Verification items for the finished model (mm, model axes). Face numbers are marked on the shaded views. A direction names the side the tool comes from. Give positions to 0.01 mm unless a question says otherwise; leave off trailing zeros. Order: outer loops, then holes, each group sorted by start corner. A loop starts at its lowest first (then second) coordinate and runs counter-clockwise, first axis right, second up. Notation, with made-up numbers: M -15.75,24.25 L 23.25,24.25 A35 ccw 23.25,63.25 Z; hole C 60,15 d8. An arc over 180 degrees is marked long. Answer as a JSON object with one key per item and string values.
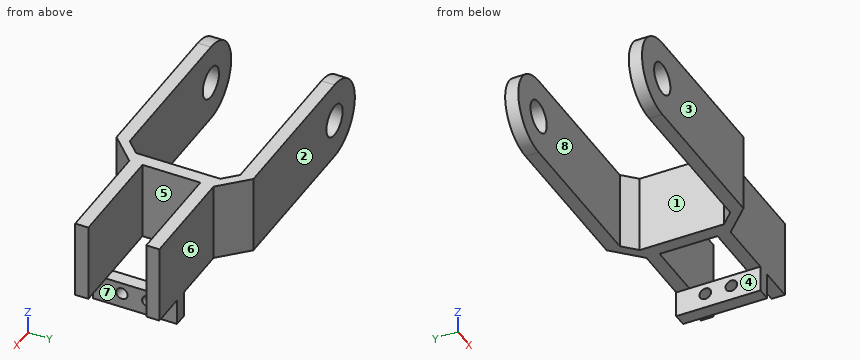
```python
from build123d import *

# Parameters (mm, degrees)
SKETCH1_R           = 6
BOSS_EXTRUDE4_DEPTH = 5
BOSS_EXTRUDE5_DEPTH = 30
BOSS_EXTRUDE6_DEPTH = 30
SKETCH11_R          = 6
BOSS_EXTRUDE7_DEPTH = 5
BOSS_EXTRUDE8_DEPTH = 30
BOSS_EXTRUDE9_DEPTH = 10
CUT_EXTRUDE2_REACH  = 126.008
SKETCH14_R          = 2.2


with BuildPart() as part:
    # Sketch1 → Boss-Extrude4 (new body)
    with BuildSketch(Plane(origin=(0, 0, 0), x_dir=(1, 0, 0), z_dir=(0, 1, 0))):
        with BuildLine():
            Line((0, 15), (60, 15))
            Line((60, 15), (60, -15))
            Line((60, -15), (0, -15))
            ThreePointArc((0, -15), (-15, 0), (0, 15))
        make_face()
        with Locations(Location((0, 0, 0), (0, 0, 270))):
            Circle(SKETCH1_R, mode=Mode.SUBTRACT)
    extrude(amount=BOSS_EXTRUDE4_DEPTH)

    # Sketch8 → Boss-Extrude5 (add)
    with BuildSketch(Plane.XY.offset(15)):
        Polygon((60, 0), (70, -10), (110, -10), (110, -5), (70, -5), (60, 5), align=None)
    extrude(amount=-BOSS_EXTRUDE5_DEPTH)

    # Sketch9 → Boss-Extrude6 (add)
    with BuildSketch(Plane.XY.offset(15)):
        Polygon((70, -10), (70, -21), (65, -21), (65, -5), align=None)
    boss_extrude6 = extrude(amount=-BOSS_EXTRUDE6_DEPTH)

    # Mirror3: Boss-Extrude6 across plane
    add(boss_extrude6.mirror(Plane(origin=(70, -21, -15), x_dir=(0, 0, 1), z_dir=(0, -1, 0))))



with BuildPart() as body_2:
    # Sketch11 → Boss-Extrude7 (new body)
    with BuildSketch(Plane(origin=(0, -42, 0), x_dir=(-1, 0, 0), z_dir=(0, -1, 0))):
        with BuildLine():
            Line((0, 15), (-60, 15))
            Line((-60, 15), (-60, -15))
            Line((-60, -15), (0, -15))
            ThreePointArc((0, -15), (15, 0), (0, 15))
        make_face()
        with Locations(Location((0, 0, 0), (0, 0, 270))):
            Circle(SKETCH11_R, mode=Mode.SUBTRACT)
    extrude(amount=BOSS_EXTRUDE7_DEPTH)


with BuildPart() as part_1:
    add(part.part)

    add(body_2.part)  # Boss-Extrude8 merges body 2
    # Sketch12 → Boss-Extrude8 (add)
    with BuildSketch(Plane(origin=(0, 0, -15), x_dir=(-1, 0, 0), z_dir=(0, 0, -1))):
        Polygon((-70, -32), (-65, -37), (-60, -42), (-60, -47), (-70, -37), (-110, -37), (-110, -32), align=None)
    extrude(amount=-BOSS_EXTRUDE8_DEPTH)

    # Sketch13 → Boss-Extrude9 (add)
    with BuildSketch(Plane(origin=(0, 0, -15), x_dir=(-1, 0, 0), z_dir=(0, 0, -1))):
        Polygon((-97, -10), (-97, -37), (-92, -37), (-92, -5), (-97, -5), align=None)
    extrude(amount=BOSS_EXTRUDE9_DEPTH)

    # Sketch14 → Cut-Extrude2 (cut, up to next)
    with BuildSketch(Plane(origin=(97, 0, 0), x_dir=(0, 0, -1), z_dir=(1, 0, 0)), mode=Mode.PRIVATE) as cut_extrude2_sk1:
        with Locations((19.3, -16.05)):
            Circle(SKETCH14_R)
    cut_extrude2_tool1 = extrude(cut_extrude2_sk1.sketch, amount=-CUT_EXTRUDE2_REACH, mode=Mode.PRIVATE) & part_1.part
    # Sketch14 → Cut-Extrude2 (cut, up to next)
    with BuildSketch(Plane(origin=(97, 0, 0), x_dir=(0, 0, -1), z_dir=(1, 0, 0)), mode=Mode.PRIVATE) as cut_extrude2_sk2:
        with Locations((19.3, -25.95)):
            Circle(SKETCH14_R)
    cut_extrude2_tool2 = extrude(cut_extrude2_sk2.sketch, amount=-CUT_EXTRUDE2_REACH, mode=Mode.PRIVATE) & part_1.part
    add(cut_extrude2_tool1.solids().sort_by_distance((97, -16.05, -19.3))[0], mode=Mode.SUBTRACT)
    add(cut_extrude2_tool2.solids().sort_by_distance((97, -25.95, -19.3))[0], mode=Mode.SUBTRACT)


solid = part_1.part
```
Q1. Section check C-C on x = 28. Record the cut outline in (y, z), then the cut area to 3 significant figures.
Resolved:
{"outline": "M -47,-15 L -42,-15 L -42,15 L -47,15 Z; M 0,-15 L 5,-15 L 5,15 L 0,15 Z", "area": "300 mm²"}
Q2. Release check for a two-part mould opening along Y. For the marked faces 1, 2 and 3 record: +Y half, -Y half, draft (parallel to the pull), parting line (faces both ways), or undercut.
Resolved:
{"face 1": "undercut", "face 2": "+Y half", "face 3": "-Y half"}
Q3. Section check D-D on z = -9. Record the cut outline in (x, y), then the cut area to 4 significant figures.
Resolved:
{"outline": "M -12,-47 L 60,-47 L 70,-37 L 110,-37 L 110,-32 L 70,-32 L 70,-10 L 110,-10 L 110,-5 L 70,-5 L 60,5 L -12,5 L -12,0 L 60,0 L 65,-5 L 65,-37 L 60,-42 L -12,-42 Z", "area": "1,355 mm²"}
Q4. Section check B-B on z = -19.3. Record the cut outline in (x, y), then the cut area to 3 significant figures.
Resolved:
{"outline": "M 92,-37 L 97,-37 L 97,-28.15 L 92,-28.15 Z; M 92,-23.75 L 97,-23.75 L 97,-18.25 L 92,-18.25 Z; M 92,-13.85 L 97,-13.85 L 97,-5 L 92,-5 Z", "area": "116 mm²"}
Q5. Material ranges on L1, parallel to Y at x = 95, z = -19; L2, parallel to Y at x = 55, z = -1; L3, parallel to Y at x = 82.5, z = -12.5, recorded low to high.
Resolved:
{"L1": "y = -37 to -28.13, -23.77 to -18.23, -13.87 to -5", "L2": "y = -47 to -42, 0 to 5", "L3": "y = -37 to -32, -10 to -5"}
Q6. Tool access check on the marked faces 4, 5, 6, 7 and 8. Record the directions out of +Z, -Z, +X, -X, +Y, -Y that give a thin tool (end or side, any length) a straight path to the whole face; none if there is none.
Resolved:
{"face 4": "-Z, -X, +Y, -Y", "face 5": "+Z, -Z, +X", "face 6": "+Z, -Z, +X, +Y", "face 7": "-Z, +X, +Y, -Y", "face 8": "+Z, -Z, -X"}
Q7. Gauge pin test, flat ends, axial feed: pin 1 Ø2 at (y, z) = (-27.5, -3.5) entering from -X; pin 2 Ø5 at (x, y) = (87, -32.5) entering from -Z; pin 3 Ø3 at (y, z) = (-23.5, -21.5) entering from +X. Record the tip position at first contact, or that the pin passes through.
Resolved:
{"pin 1": "stops at x = 65", "pin 2": "stops at z = -15", "pin 3": "stops at x = 97"}
Q8. Section check A-A on y = -16.05. Record the cut outline in (x, z).
Resolved:
{"outline": "M 65,-15 L 70,-15 L 70,15 L 65,15 Z; M 92,-25 L 97,-25 L 97,-21.5 L 92,-21.5 Z; M 92,-17.1 L 97,-17.1 L 97,-15 L 92,-15 Z"}
